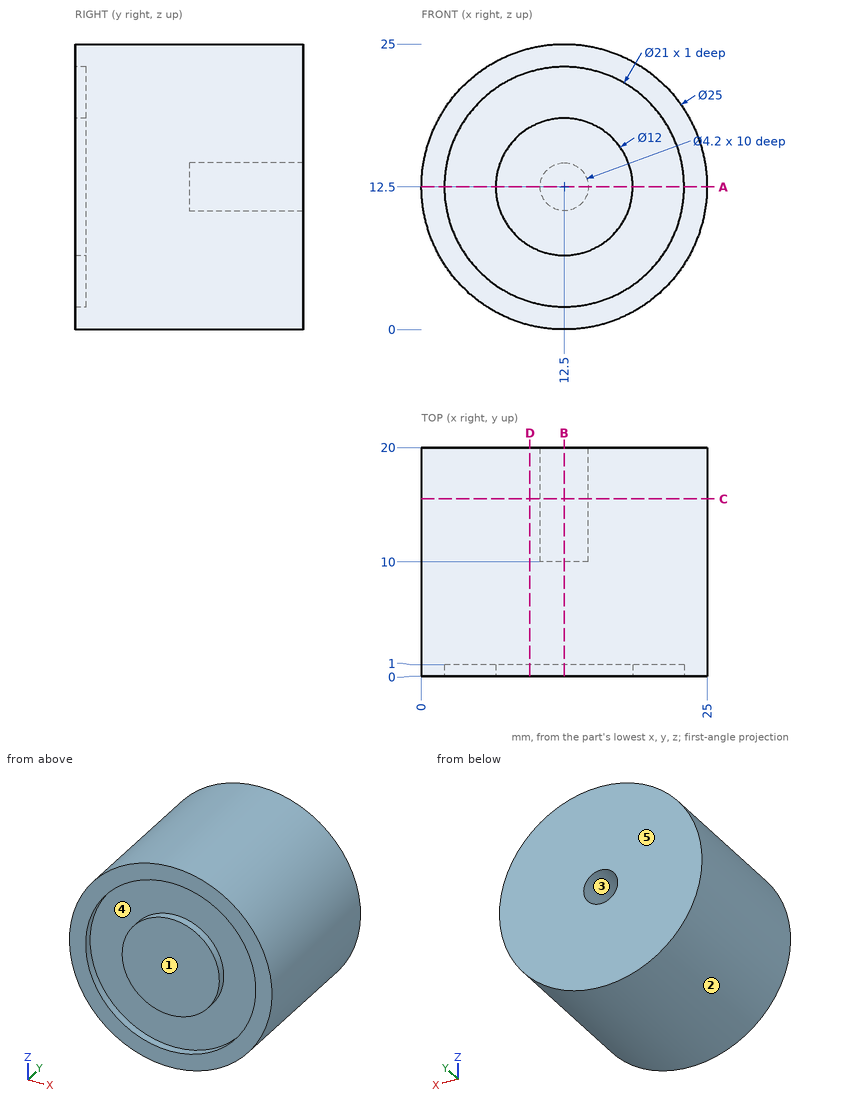
For this review, use the dimensioned drawing (mm, ordinates from the lowest corner) and the shaded views. A direction names the side the tool comes from. Give positions to 0.01 mm unless a question says otherwise; leave off trailing zeros. Loops run counter-clockwise (first coordinate to the right, second up) from the corner with the lowest first, then second, coordinate; pieces in that order, holes last. Notation, with made-up numbers: (-38, 82) -> (11, 82) arc R19 cw to (11, 96) -> close; hole circle Ø7 at (52, 11). An arc over 180 degrees is marked (long way). Use CSV: the item, a comma, the result in double quotes.
1. Consider section A-A, the plane z = 12.5. Write out the cut boundary in (x, y).
Result:
outline,"(0, 0) -> (2, 0) -> (2, 1) -> (6.5, 1) -> (6.5, 0) -> (18.5, 0) -> (18.5, 1) -> (23, 1) -> (23, 0) -> (25, 0) -> (25, 20) -> (14.6, 20) -> (14.6, 10) -> (10.4, 10) -> (10.4, 20) -> (0, 20) -> close"
2. For P1, Ø4, axis at y = 5, z = 22, coming from the -X side; P2, Ø2, axis at x = 12, z = 13, coming from the +Y side; P3, Ø6, axis at y = 10.5, z = 19.5, coming from the +X side, all flat-tipped, find the tip position at first contact; note any pin that passes through.
Result:
P1,"stops at x = 2.5"
P2,"stops at y = 10"
P3,"stops at x = 24.34"
3. The part is to be moulded in two halves that separate along X. For the marked faces 1, 2 and 3, say which applies: +X half, -X half, draft (parallel to the pull), parting line (faces both ways), or undercut.
Result:
face 1,"draft"
face 2,"parting line"
face 3,"undercut"
4. Consider section D-D, the plane x = 9.5. Write out the cut boundary in (y, z), then the cut area to 3 significant figures.
Result:
outline,"(0, 0.37) -> (20, 0.37) -> (20, 24.63) -> (0, 24.63) -> (0, 22.56) -> (1, 22.56) -> (1, 17.7) -> (0, 17.7) -> (0, 7.3) -> (1, 7.3) -> (1, 2.44) -> (0, 2.44) -> close"
area,"476 mm²"
5. Consider section C-C, the plane y = 15.5. Write out the cut boundary in (x, z).
Result:
outline,"circle Ø25 at (12.5, 12.5); hole circle Ø4.2 at (12.5, 12.5)"
6. Consider section B-B, the plane x = 12.5. Write out the cut boundary in (y, z).
Result:
outline,"(0, 0) -> (20, 0) -> (20, 10.4) -> (10, 10.4) -> (10, 14.6) -> (20, 14.6) -> (20, 25) -> (0, 25) -> (0, 23) -> (1, 23) -> (1, 18.5) -> (0, 18.5) -> (0, 6.5) -> (1, 6.5) -> (1, 2) -> (0, 2) -> close"
7. Machinability: for the marked faces 4 and 5, which of the approach directions +Z, -Z, +X, -X, +Y, -Y give a long, thin tool a straight path to every point of the face, cutting with its end or side? Answer none if there is none.
Result:
face 4,"-Y"
face 5,"+Z, -Z, +X, -X, +Y"
8. To check wall thickness, follow probe 1 along X at (y, z) = (0.3, 12.5); probe 2 along X at (y, z) = (13.75, 12.5); probe 3 along Y at (x, z) = (2.25, 13.25). State the ranges of each line that lie inside material, in increasing order. Write a range as from..to.
Result:
probe 1,"x = 0..2, 6.5..18.5, 23..25"
probe 2,"x = 0..10.4, 14.6..25"
probe 3,"y = 1..20"
